```python
from build123d import *

# Parameters (mm, degrees)
BOSS_EXTRUDE1_DEPTH = 31
SKETCH3_R           = 12.5
CUT_EXTRUDE1_DEPTH  = 87.208303263
SKETCH4_W           = 31
SKETCH4_H           = 15
BOSS_EXTRUDE2_DEPTH = 11
SKETCH5_W           = 31
SKETCH5_H           = 10
BOSS_EXTRUDE3_DEPTH = 56
SKETCH6_R           = 1.4
BOSS_EXTRUDE4_DEPTH = 10
SKETCH7_W           = 31
SKETCH7_H           = 15
BOSS_EXTRUDE5_DEPTH = 16
SKETCH8_W           = 31
SKETCH8_H           = 10
BOSS_EXTRUDE6_DEPTH = 9
FILLET1_R           = 4


with BuildPart() as part:
    # Sketch1 → Boss-Extrude1 (new body)
    with BuildSketch(Plane.XY):
        with BuildLine():
            Line((-15.5, 107.5), (-15.5, 28.565713714))
            ThreePointArc((-15.5, 28.565713714), (0, 32.5), (15.5, 28.565713714))
            Line((15.5, 28.565713714), (15.5, 107.5))
            Line((15.5, 107.5), (-15.5, 107.5))
        make_face()
    extrude(amount=BOSS_EXTRUDE1_DEPTH)

    # Sketch3 → Cut-Extrude1 (cut, through all)
    with BuildSketch(Plane(origin=(0, 107.5, 0), x_dir=(1, 0, 0), z_dir=(0, 1, 0))):
        with Locations(Location((0, -15.5, 0), (0, 0, 270))):
            Circle(SKETCH3_R)
    extrude(amount=-CUT_EXTRUDE1_DEPTH, mode=Mode.SUBTRACT)

    # Sketch4 → Boss-Extrude2 (add)
    with BuildSketch(Plane.XY.offset(31)):
        with Locations((0, 36.065713714)):
            Rectangle(SKETCH4_W, SKETCH4_H)
    extrude(amount=BOSS_EXTRUDE2_DEPTH)

    # Sketch5 → Boss-Extrude3 (add)
    with BuildSketch(Plane.XZ.offset(-28.565713714)):
        with Locations((0, 37)):
            Rectangle(SKETCH5_W, SKETCH5_H)
    extrude(amount=BOSS_EXTRUDE3_DEPTH)

    # Sketch6 → Boss-Extrude4 (add)
    with BuildSketch(Plane.XZ.offset(27.434286286)):
        with Locations(Location((-10, 37.5, 0), (0, 0, 270))):
            Circle(SKETCH6_R)
        with Locations(Location((10, 37.5, 0), (0, 0, 270))):
            Circle(SKETCH6_R)
    extrude(amount=BOSS_EXTRUDE4_DEPTH)

    # Sketch7 → Boss-Extrude5 (add)
    with BuildSketch(Plane(origin=(0, 0, 0), x_dir=(-1, 0, 0), z_dir=(0, 0, -1))):
        with Locations((0, 36.065713714)):
            Rectangle(SKETCH7_W, SKETCH7_H)
    extrude(amount=BOSS_EXTRUDE5_DEPTH)

    # Sketch8 → Boss-Extrude6 (add)
    with BuildSketch(Plane.XZ.offset(-28.565713714)):
        with Locations((0, -11)):
            Rectangle(SKETCH8_W, SKETCH8_H)
    extrude(amount=BOSS_EXTRUDE6_DEPTH)

    # Fillet1
    fillet1_edges = [part.edges().sort_by_distance(p)[0] for p in [
        (0, 43.565713714, 31),
        (0, 43.565713714, 0),
    ]]
    fillet(fillet1_edges, radius=FILLET1_R)


solid = part.part
```
Input: part model. Units: mm. Frame: model coordinates. A direction names the side the tool comes from. Give positions to 0.01 mm unless a question says otherwise; leave off trailing zeros. Order: outer loops, then holes, each group sorted by start corner. A loop starts at its lowest first (then second) coordinate and runs counter-clockwise, first axis right, second up. Notation, with made-up numbers: (57, 30.5) - (102, 30.5) arc R23 cw to (102, 43.5) - close; hole circle Ø6 at (-37.75, 64). An arc over 180 degrees is marked (long way). One line per item, written item: value.
1. Draft query along Z for faces 4 (the face through (7.1, 107.5, 4.9)), 5 (the face through (8.45, 69.29, 6.29)), 6 (the face through (0.22, 44.77, 32.14)). Return one class per face: released by +Z, released by -Z, zero draft, split by the parting line, or undercut.
Determined:
face 4: zero draft
face 5: undercut
face 6: released by +Z
2. Cut plane D-D, the plane z = 37.5. Output: boundary loops of the cut face in (x, y).
Determined:
outline: (-15.5, -27.43) - (-11.4, -27.43) - (-11.4, -37.43) - (-8.6, -37.43) - (-8.6, -27.43) - (8.6, -27.43) - (8.6, -37.43) - (11.4, -37.43) - (11.4, -27.43) - (15.5, -27.43) - (15.5, 43.57) - (-15.5, 43.57) - close
3. Cut plane C-C, the plane y = 62. Output: boundary loops of the cut face in (x, z).
Determined:
outline: (-15.5, 0) - (15.5, 0) - (15.5, 31) - (-15.5, 31) - close; hole circle Ø25 at (0, 15.5)
4. Cut plane A-A, the plane z = 15.5. Output: boundary loops of the cut face in (x, y).
Determined:
outline: (-15.5, 28.57) arc R32.5 cw to (-12.5, 30) - (-12.5, 107.5) - (-15.5, 107.5) - close; (12.5, 30) arc R32.5 cw to (15.5, 28.57) - (15.5, 107.5) - (12.5, 107.5) - close
5. Reachability of faces 1 (the face through (0, 19.566, -11)), 2 (the face through (0, 30, 31)), 3 (the face through (0, 78, 0)) from +Z, -Z, +X, -X, +Y, -Y: full face, straight path, thin tool, end or side. Return the list, or none.
Determined:
face 1: -Z, +X, -X, -Y
face 2: -Y
face 3: -Z, +X, -X, +Y
6. Pin query (flat end, axial travel): pin 1 Ø2 at (y, z) = (-19.5, 30) entering from -X; pin 2 Ø5 at (x, z) = (-4.5, -11) entering from -Y; pin 3 Ø9.5 at (x, y) = (-0.5, 63.5) entering from -Z; pin 4 Ø1.5 at (x, z) = (5, 27.5) entering from -Y. Return the tip coordinate at first contact, or that it passes through.
Determined:
pin 1: through
pin 2: y = 19.57
pin 3: z = 0
pin 4: y = 31.99
7. Cut plane B-B, the plane x = 0. Output: boundary loops of the cut face in (y, z).
Determined:
outline: (-27.43, 32) - (28.57, 32) - (28.57, 31) - (32.5, 31) - (32.5, 28) - (107.5, 28) - (107.5, 31) - (47.57, 31) arc R4 cw to (43.57, 35) - (43.57, 42) - (-27.43, 42) - close; (19.57, -16) - (43.57, -16) - (43.57, -4) arc R4 cw to (47.57, 0) - (107.5, 0) - (107.5, 3) - (32.5, 3) - (32.5, 0) - (28.57, 0) - (28.57, -6) - (19.57, -6) - close
8. Line query: probe 1 along Z at (x, y) = (0, 83.5); probe 2 along X at (y, z) = (63, 15.5); probe 3 along Y at (x, z) = (7, -7). Output: solid intervals per line, ascending.
Determined:
probe 1: 0 to 3, 28 to 31
probe 2: -15.5 to -12.5, 12.5 to 15.5
probe 3: 19.57 to 43.57
